from build123d import *

# Parameters (mm, degrees)
F_3_8_CLEARANCE_HOLE1_D                = 10.0838
CIRPATTERN1_COUNT                      = 10
F_3_8_0_375_DIAMETER_HOLE1_D           = 9.525
F_1_4_0_25_DIAMETER_HOLE1_D            = 6.35
CUT_EXTRUDE1_DEPTH                     = 108.882743755
CUT_EXTRUDE1_DEPTH_BACK                = 108.882743755
SKETCH7_R                              = 0.635
F_1_8_0_125_DIAMETER_HOLE1_D           = 3.175
F_1_8_0_125_DIAMETER_HOLE1_CSINK_D     = 3.81
F_1_8_0_125_DIAMETER_HOLE1_CSINK_ANGLE = 90


with BuildPart() as part:
    # Sketch1 → Revolve1 (revolve)
    with BuildSketch(Plane.XY, mode=Mode.PRIVATE) as revolve1_sk:
        Polygon((0, 0), (0, -5.08), (54.8259, -5.08), (54.8259, -2.3876), (58.8899, -2.3876), (58.8899, -5.08), (76.2, -5.08), (76.2, 0), align=None)
    revolve(revolve1_sk.sketch.rotate(Axis((0, 0, 0), (0, -1, 0)), 90), axis=Axis((0, 0, 0), (0, -1, 0)))

    # 3/8 Clearance Hole1 (through all)
    with Locations(Plane(origin=(67.31, 0, 0), x_dir=(0, 0, 1), z_dir=(0, 1, 0))):
        with Locations((0, 0)):
            f_3_8_clearance_hole1 = Hole(F_3_8_CLEARANCE_HOLE1_D / 2)

    # CirPattern1: 3/8 Clearance Hole1 ×10 about axis
    cirpattern1_axis = Axis((0, 0, 0), (0, 1, 0))
    for i in range(1, CIRPATTERN1_COUNT):
        add(f_3_8_clearance_hole1.rotate(cirpattern1_axis, i * 360 / CIRPATTERN1_COUNT), mode=Mode.SUBTRACT)

    # 3/8 (0.375) Diameter Hole1 (through all)
    with Locations(Plane(origin=(44.45, 0, 0), x_dir=(0, 0, 1), z_dir=(0, 1, 0))):
        with Locations((0, 0), (0, -88.9)):
            Hole(F_3_8_0_375_DIAMETER_HOLE1_D / 2)

    # 1/4 (0.25) Diameter Hole1 (through all)
    with Locations(Plane(origin=(-25.4, 0, -38.1), x_dir=(0, 0, 1), z_dir=(0, 1, 0))):
        with Locations((0, 0)):
            Hole(F_1_4_0_25_DIAMETER_HOLE1_D / 2)

    # Sketch7 → Cut-Extrude1 (cut, two sides: drawn at the far end of the back side and taken through both)
    with BuildSketch(Plane(origin=(0, 0, 0), x_dir=(1, 0, 0), z_dir=(0, 1, 0)).offset(-CUT_EXTRUDE1_DEPTH_BACK)):
        with Locations(Location((10.3632, 0, 0), (0, 0, 270))):
            Circle(SKETCH7_R)
        with Locations(Location((18.2118, 0, 0), (0, 0, 270))):
            Circle(SKETCH7_R)
        with Locations(Location((24.511, 0, 0), (0, 0, 270))):
            Circle(SKETCH7_R)
        with Locations(Location((5.1816, -8.974794464, 0), (0, 0, 270))):
            Circle(SKETCH7_R)
        with Locations(Location((-5.1816, -8.974794464, 0), (0, 0, 270))):
            Circle(SKETCH7_R)
        with Locations(Location((-10.3632, 0, 0), (0, 0, 270))):
            Circle(SKETCH7_R)
        with Locations(Location((-5.1816, 8.974794464, 0), (0, 0, 270))):
            Circle(SKETCH7_R)
        with Locations(Location((5.1816, 8.974794464, 0), (0, 0, 270))):
            Circle(SKETCH7_R)
        with Locations(Location((15.771881449, -9.1059, 0), (0, 0, 270))):
            Circle(SKETCH7_R)
        with Locations(Location((9.1059, -15.771881449, 0), (0, 0, 270))):
            Circle(SKETCH7_R)
        with Locations(Location((0, -18.2118, 0), (0, 0, 270))):
            Circle(SKETCH7_R)
        with Locations(Location((-9.1059, -15.771881449, 0), (0, 0, 270))):
            Circle(SKETCH7_R)
        with Locations(Location((-15.771881449, -9.1059, 0), (0, 0, 270))):
            Circle(SKETCH7_R)
        with Locations(Location((-18.2118, 0, 0), (0, 0, 270))):
            Circle(SKETCH7_R)
        with Locations(Location((-15.771881449, 9.1059, 0), (0, 0, 270))):
            Circle(SKETCH7_R)
        with Locations(Location((-9.1059, 15.771881449, 0), (0, 0, 270))):
            Circle(SKETCH7_R)
        with Locations(Location((0, 18.2118, 0), (0, 0, 270))):
            Circle(SKETCH7_R)
        with Locations(Location((9.1059, 15.771881449, 0), (0, 0, 270))):
            Circle(SKETCH7_R)
        with Locations(Location((15.771881449, 9.1059, 0), (0, 0, 270))):
            Circle(SKETCH7_R)
        with Locations(Location((23.675807928, -6.343913615, 0), (0, 0, 270))):
            Circle(SKETCH7_R)
        with Locations(Location((21.227148672, -12.2555, 0), (0, 0, 270))):
            Circle(SKETCH7_R)
        with Locations(Location((17.331894314, -17.331894314, 0), (0, 0, 270))):
            Circle(SKETCH7_R)
        with Locations(Location((12.2555, -21.227148672, 0), (0, 0, 270))):
            Circle(SKETCH7_R)
        with Locations(Location((6.343913615, -23.675807928, 0), (0, 0, 270))):
            Circle(SKETCH7_R)
        with Locations(Location((0, -24.511, 0), (0, 0, 270))):
            Circle(SKETCH7_R)
        with Locations(Location((-6.343913615, -23.675807928, 0), (0, 0, 270))):
            Circle(SKETCH7_R)
        with Locations(Location((-12.2555, -21.227148672, 0), (0, 0, 270))):
            Circle(SKETCH7_R)
        with Locations(Location((-17.331894314, -17.331894314, 0), (0, 0, 270))):
            Circle(SKETCH7_R)
        with Locations(Location((-21.227148672, -12.2555, 0), (0, 0, 270))):
            Circle(SKETCH7_R)
        with Locations(Location((-23.675807928, -6.343913615, 0), (0, 0, 270))):
            Circle(SKETCH7_R)
        with Locations(Location((-24.511, 0, 0), (0, 0, 270))):
            Circle(SKETCH7_R)
        with Locations(Location((-23.675807928, 6.343913615, 0), (0, 0, 270))):
            Circle(SKETCH7_R)
        with Locations(Location((-21.227148672, 12.2555, 0), (0, 0, 270))):
            Circle(SKETCH7_R)
        with Locations(Location((-17.331894314, 17.331894314, 0), (0, 0, 270))):
            Circle(SKETCH7_R)
        with Locations(Location((-12.2555, 21.227148672, 0), (0, 0, 270))):
            Circle(SKETCH7_R)
        with Locations(Location((-6.343913615, 23.675807928, 0), (0, 0, 270))):
            Circle(SKETCH7_R)
        with Locations(Location((0, 24.511, 0), (0, 0, 270))):
            Circle(SKETCH7_R)
        with Locations(Location((6.343913615, 23.675807928, 0), (0, 0, 270))):
            Circle(SKETCH7_R)
        with Locations(Location((12.2555, 21.227148672, 0), (0, 0, 270))):
            Circle(SKETCH7_R)
        with Locations(Location((17.331894314, 17.331894314, 0), (0, 0, 270))):
            Circle(SKETCH7_R)
        with Locations(Location((21.227148672, 12.2555, 0), (0, 0, 270))):
            Circle(SKETCH7_R)
        with Locations(Location((23.675807928, 6.343913615, 0), (0, 0, 270))):
            Circle(SKETCH7_R)
    extrude(amount=CUT_EXTRUDE1_DEPTH + CUT_EXTRUDE1_DEPTH_BACK, mode=Mode.SUBTRACT)

    # 1/8 (0.125) Diameter Hole1 (through all)
    with Locations(Plane(origin=(0, 0, 45.72), x_dir=(0, 0, 1), z_dir=(0, 1, 0))):
        with Locations((0, 0), (-91.44, 0)):
            CounterSinkHole(F_1_8_0_125_DIAMETER_HOLE1_D / 2, F_1_8_0_125_DIAMETER_HOLE1_CSINK_D / 2, counter_sink_angle=F_1_8_0_125_DIAMETER_HOLE1_CSINK_ANGLE)


solid = part.part
Input: part model. Units: mm. Frame: model coordinates. A direction names the side the tool comes from. Coordinates: 2 decimals unless noted, no trailing zeros. Loops run counter-clockwise (first coordinate to the right, second up) from the corner with the lowest first, then second, coordinate; pieces in that order, holes last. Notation, with made-up numbers: (67.25, -26.5) - (101.25, -26.5) arc R10 ccw to (101.25, -8.5) - close; hole circle Ø5 at (1, 56). An arc over 180 degrees is marked (long way). Answer in a Markdown table with one row per item. Add a question column.
Item 1: Line query: line 1 along Z through (x, y) = (32, -4.8); line 2 along Z through (x, y) = (28.5, -4.65); line 3 along X through (y, z) = (-4.5, -40.5). Output: solid intervals per line, ascending. Write a range as [from, to].
Item 2: Section query C-C on y = -3.3. State how many separate pieces and enclosed holes the cut face has, then the cut area to 3 significant figures.
Item 3: Section query D-D on z = -37.5. Return the cut outline in (x, y).
Item 4: Access query for faces 5 (the cylindrical face through (52.853, -2.576, -44.345)), 6 (the cylindrical face through (33.36, -3.71, -43.51)). Directions: +Z, -Z, +X, -X, +Y, -Y. A direction counts if a zero-diameter tool reaches every point of the face in a straight line with its end or side. Return the directions, or none.
Item 5: Contact query for flat-ended pins moving along their axis: P1, Ø2, axis at x = 7, y = -3.5, coming from the +Z side; P2, Ø0.8, axis at x = 15.77, z = 9.11, coming from the -Y side; P3, Ø3, axis at x = 46, y = -4, coming from the -Z side; P4, Ø1, axis at x = -49.5, y = -3, coming from the -Z side. Output: stop coordinate, or through.
Item 6: Section query B-B on x = 67.31. Return the cut outline in (y, z).
Item 7: Mould query, pull axis Z, two halves, no side actions, for faces 1 (the cylindrical face through (-23.254, -2.576, -35.76)), 2 (the cylindrical face through (74.388, -2.504, -16.519)), 3 (the cylindrical face through (39.8, -2.58, 1.03)), 4 (the flat face through (-57, -5.08, 17)). Classes: released by +Z, released by -Z, zero draft, split by the parting line, or undercut.
Item 8: Section query A-A on z = 40.5. Return the cut outline in (x, y).
Recorded:
| question | item | result |
|---|---|---|
| 1 | line 1 | [-69.16, -49.44], [-44.52, 44.52], [49.44, 69.16] |
| 1 | line 2 | [-70.67, -51.53], [-46.84, 46.84], [51.53, 70.67] |
| 1 | line 3 | [-64.55, -59.41], [-49.5, -42.75], [-36.95, -27.48], [-23.32, 36.95], [42.75, 49.5], [59.41, 64.55] |
| 2 | separate pieces | 2 |
| 2 | enclosed holes | 58 |
| 2 | area | 15,700 mm^2 |
| 3 | outline | (-66.33, -5.08) - (-59.06, -5.08) - (-59.06, 0) - (-66.33, 0) - close; (-49.85, -5.08) - (-45.41, -5.08) - (-45.41, -2.39) - (-40, -2.39) - (-40, -5.08) - (-28.52, -5.08) - (-28.52, 0) - (-49.85, 0) - close; (-22.28, -5.08) - (40, -5.08) - (40, -2.39) - (45.41, -2.39) - (45.41, -5.08) - (49.85, -5.08) - (49.85, 0) - (-22.28, 0) - close; (59.06, -5.08) - (66.33, -5.08) - (66.33, 0) - (59.06, 0) - close |
| 4 | face 5 | +Y, -Y |
| 4 | face 6 | -Y |
| 5 | P1 | z = 75.96 |
| 5 | P2 | through |
| 5 | P3 | z = -61.86 |
| 5 | P4 | z = -58.36 |
| 6 | outline | (-5.08, -35.72) - (0, -35.72) - (0, -5.04) - (-5.08, -5.04) - close; (-5.08, 5.04) - (0, 5.04) - (0, 35.72) - (-5.08, 35.72) - close |
| 7 | face 1 | undercut |
| 7 | face 2 | split by the parting line |
| 7 | face 3 | undercut |
| 7 | face 4 | zero draft |
| 8 | outline | (-64.55, -5.08) - (-59.41, -5.08) - (-59.41, 0) - (-64.55, 0) - close; (-49.5, -5.08) - (-42.75, -5.08) - (-42.75, -2.39) - (-36.95, -2.39) - (-36.95, -5.08) - (36.95, -5.08) - (36.95, -2.39) - (42.75, -2.39) - (42.75, -5.08) - (49.5, -5.08) - (49.5, 0) - (-49.5, 0) - close; (59.41, -5.08) - (64.55, -5.08) - (64.55, 0) - (59.41, 0) - close |
